```python
from build123d import *

# Parameters (mm, degrees)
SKETCH1_W           = 152.4
SKETCH1_H           = 152.4
SKETCH1_R           = 59.69
BOSS_EXTRUDE1_DEPTH = 0.4191
SKETCH2_R           = 2.54
CUT_EXTRUDE1_DEPTH  = 108.766333236
CIRPATTERN1_COUNT   = 4


with BuildPart() as part:
    # Sketch1 → Boss-Extrude1 (new, symmetric)
    with BuildSketch(Plane(origin=(0, 0, 0), x_dir=(1, 0, 0), z_dir=(0, 1, 0))):
        Rectangle(SKETCH1_W, SKETCH1_H)
        with Locations(Location((0, 0, 0), (0, 0, 270))):
            Circle(SKETCH1_R, mode=Mode.SUBTRACT)
    extrude(amount=BOSS_EXTRUDE1_DEPTH, both=True)

    # Sketch2 → Cut-Extrude1 (cut, through all)
    with BuildSketch(Plane(origin=(0, 0.4191, 0), x_dir=(1, 0, 0), z_dir=(0, 1, 0))):
        with Locations(Location((-60.96, 60.96, 0), (0, 0, 270))):
            Circle(SKETCH2_R)
    cut_extrude1 = extrude(amount=-CUT_EXTRUDE1_DEPTH, mode=Mode.SUBTRACT)

    # CirPattern1: Cut-Extrude1 ×4 about axis
    cirpattern1_axis = Axis((0, 0, 0), (0, 1, 0))
    for i in range(1, CIRPATTERN1_COUNT):
        add(cut_extrude1.rotate(cirpattern1_axis, i * 360 / CIRPATTERN1_COUNT), mode=Mode.SUBTRACT)


solid = part.part
```
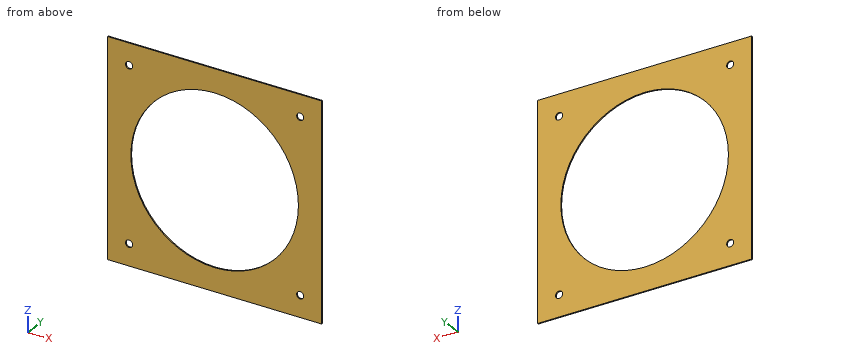
Check sheet for the modelled part. Datum: model origin and axes. Units: mm. Give positions to 0.01 mm unless a question says otherwise; leave off trailing zeros. Write each loop counter-clockwise with the first axis right and the second up, starting at its lowest first coordinate (ties: lowest second). Pieces come first, ordered by that corner, then holes. Notation, with made-up numbers: (83.25, 3.5) - (115.25, 3.5) arc R25 ccw to (115.25, 42.5) - close; hole circle Ø11 at (44, -1.5). An arc over 180 degrees is marked (long way). Answer as a JSON object with one key per item and string values. Group by question number.
1) Sectioned sample at B-B (x = 0). Record the cut outline in (y, z).
2) Sectioned sample at A-A (z = 0). Record the cut outline in (x, y).
3) Sectioned sample at C-C (y = 0.25). Record the cut outline in (x, z), then the cut area to 3 significant figures.
4) Depth check by flat-ended pin: P1, Ø4.5, axis at x = 60.96, z = 60.96, coming from the +Y side. Enter the tip coordinate at first touch or a pass-through.
5) Thickness scan on probe 1 along X at (y, z) = (0.25, 60.96); probe 2 along Z at (x, y) = (-62, -0.1). Record the ranges inside material, lowest first. Write a range as from..to.
Geometry results:
{
 "1": {"outline": "(-0.42, -76.2) - (0.42, -76.2) - (0.42, -59.69) - (-0.42, -59.69) - close; (-0.42, 59.69) - (0.42, 59.69) - (0.42, 76.2) - (-0.42, 76.2) - close"},
 "2": {"outline": "(-76.2, -0.42) - (-59.69, -0.42) - (-59.69, 0.42) - (-76.2, 0.42) - close; (59.69, -0.42) - (76.2, -0.42) - (76.2, 0.42) - (59.69, 0.42) - close"},
 "3": {"outline": "(-76.2, -76.2) - (76.2, -76.2) - (76.2, 76.2) - (-76.2, 76.2) - close; hole circle Ø5.08 at (-60.96, -60.96); hole circle Ø5.08 at (-60.96, 60.96); hole circle Ø119.38 at (0, 0); hole circle Ø5.08 at (60.96, -60.96); hole circle Ø5.08 at (60.96, 60.96)", "area": "12,000 mm^2"},
 "4": {"P1": "passes through"},
 "5": {"probe 1": "x = -76.2..-63.5, -58.42..58.42, 63.5..76.2", "probe 2": "z = -76.2..-63.28, -58.64..58.64, 63.28..76.2"}
}
